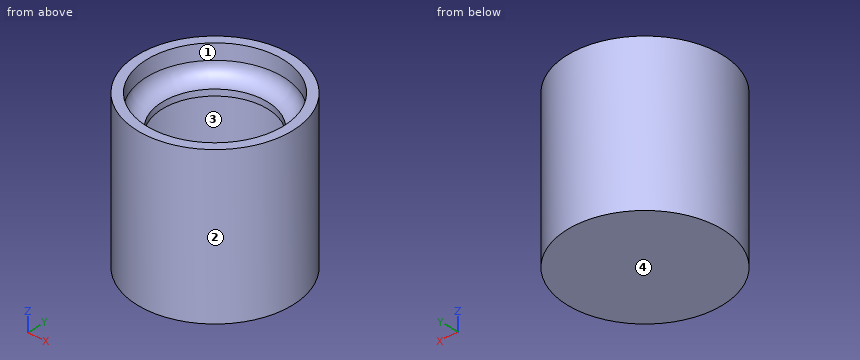
from build123d import *

# Parameters (mm, degrees)
F0_R     = 25
F1_DEPTH = 50
F2_R     = 22
F3_DEPTH = 10
F4_R     = 5
F5_T     = 2


# Not quite as in the source:
# - a shell that OpenCascade refuses in one call is made with other operations: the cavity is built on its own and cut out


with BuildPart() as f1:
    # F0 (on Top) → F1 (new body)
    with BuildSketch(Plane.XY):
        Circle(F0_R)
    extrude(amount=F1_DEPTH)

    # F2 (on face) → F3 (cut)
    with BuildSketch(Plane.XY.offset(50)):
        Circle(F2_R)
    extrude(amount=-F3_DEPTH, mode=Mode.SUBTRACT)

    # F4
    f4_edges = [f1.edges().sort_by_distance(p)[0] for p in [
        (-22, 0, 40),
    ]]
    fillet(f4_edges, radius=F4_R)

    # F5: shell of thickness 2, made by hand


with BuildPart() as f5_core1:
    # F5_t2: copy of F1
    add(f1.part)

    # the walls: a layer under each face that stays
    f5_faces = [f5_core1.faces().sort_by_distance(p)[0] for p in [
        (-22, 0, 47.5),
        (-20.5355339059, 0, 41.4644660941),
        (-16.6666666667, -16.6666666667, 50),
        (-25, 0, 25),
        (0, 0, 0),
    ]]
    thicken(f5_faces, amount=-F5_T, mode=Mode.SUBTRACT)


with BuildPart() as f1_1:
    add(f1.part)

    # what is left inside the walls is the cavity
    f5_cavity = [f5_core1.part.solids().sort_by_distance(p)[0] for p in [
        (-22.98, 0, 28.262966),
    ]]
    add(f5_cavity, mode=Mode.SUBTRACT)


solid = f1_1.part
Verification items for the finished model (mm, model axes). Face numbers are marked on the shaded views. Give positions to 0.01 mm unless a question says otherwise; leave off trailing zeros. Write each loop counter-clockwise with the first axis right and the second up, starting at its lowest first coordinate (ties: lowest second). Pieces come first, ordered by that corner, then holes. Notation, with made-up numbers: M 69.25,13.5 L 74.25,13.5 A14 cw 74.25,18.5 Z; hole C -26,-28.5 d3. An arc over 180 degrees is marked long. Write item = value, one per line.
(1) Sectioned sample at B-B (z = 6). Record the cut outline in (x, y), then the cut area to 3 significant figures.
Found:
outline = C 0,0 d50; hole C 0,0 d46
area = 302 mm2
(2) Draft check along X on the marked faces 1, 2, 3 and 4. Enter one of: released by +X, released by -X, zero draft, split by the parting line, or undercut.
Found:
face_1 = undercut
face_2 = split by the parting line
face_3 = undercut
face_4 = zero draft
(3) Material ranges on line 1 (Z direction, x = 6, y = -16); line 2 (Z direction, x = -16.5, y = 1); line 3 (Y direction, x = 3, z = 43.5), recorded low to high.
Found:
line_1 = 0 to 2, 38 to 40
line_2 = 0 to 2
line_3 = -24.82 to -21.56, 21.56 to 24.82
(4) Sectioned sample at A-A (y = 0). Record the cut outline in (x, z), then the cut area to 3 significant figures.
Found:
outline = M -25,0 L 25,0 L 25,50 L 22,50 L 22,45 A5 cw 17,40 L 17,38 A7 ccw 23,41.39 L 23,2 L -23,2 L -23,41.39 A7 ccw -17,38 L -17,40 A5 cw -22,45 L -22,50 L -25,50 Z
area = 335 mm2
(5) Go/stop test with flat-tipped pins: pin 1 Ø3 at (y, z) = (5.5, 39) entering from +X; pin 2 Ø4 at (y, z) = (10, 23.5) entering from -X; pin 3 Ø2 at (x, z) = (10, 35.5) entering from +Y. Record where each tip stops, or that it passes through.
Found:
pin_1 = 24.68
pin_2 = -23.69
pin_3 = 23.32
